Autodesk Inventor part; units mm, degrees
ref_plane "YZ Plane" through (0, 0, 0) normal (1, 0, 0) x (0, 1, 0)
ref_plane "XZ Plane" through (0, 0, 0) normal (0, 1, 0) x (-1, 0, 0)
ref_plane "XY Plane" through (0, 0, 0) normal (0, 0, 1) x (1, 0, 0)
sketch "Sketch1" plane through (0, 0, 0) normal (0, 1, 0) x (-1, 0, 0)
  line L0 (-5.5, -12) -> (5.5, -12)
  line L1 (5.5, -12) -> (5.5, 12)
  line L2 (5.5, 12) -> (-5.5, 12)
  line L3 (-5.5, 12) -> (-5.5, -12)
  line L4 (-5.5, -12) -> (5.5, 12) construction
  line L5 (5.5, -12) -> (-5.5, 12) construction
  point P0 (0, 0)
  dimension "d0" = 11
  dimension "d1" = 24
extrude "Extrusion1" add sketch "Sketch1" along normal blind 10
shell "Shell1" thickness 1 removed faces 1 at (1.8333, 10, 4)
sketch "Sketch2" plane through (-5.5, 0, 12) normal (0, 0, 1) x (1, 0, 0)
  line L0 (0, 10) -> (11, 10)
  circle A0 centre (5.5, 6.75) radius 3.5
  point P0 (5.5, 0)
  point P1 (4.201, 10)
  point P2 (6.799, 10)
  dimension "d5" = 7
  dimension "d6" = 0.25
extrude "Extrusion2" cut sketch "Sketch2" against normal blind 9 contours L0 A0 picked at (4.7002, 5.9949)
sketch "Sketch3" plane through (0, 10, 0) normal (0, 1, 0) x (1, 0, 0)
  line L0 (1.299, -12) -> (5.5, -12)
  line L1 (5.5, -12) -> (5.5, 12)
  line L2 (5.5, 12) -> (-5.5, 12)
  line L3 (-5.5, 12) -> (-5.5, -12)
  line L4 (-5.5, -12) -> (-1.299, -12)
  line L5 (-5.5, 12) -> (5.5, 12)
  line L6 (5.5, 12) -> (5.5, -12)
  line L7 (5.5, -12) -> (-5.5, -12)
  line L8 (-5.5, -12) -> (-5.5, 12)
  point P0 (0, 0)
  point P1 (-1.299, -12)
extrude "Extrusion3" add sketch "Sketch3" along normal blind 1
sketch "Sketch5" plane through (0, 0, 0) normal (0, -1, 0) x (1, 0, 0)
  line L0 (4.5, -11) -> (-4.5, -11)
  line L1 (3, -11) -> (-3, -11)
  line L2 (-3, -11) -> (-3, -6.5)
  line L3 (-2.25, -5.75) -> (2.25, -5.75)
  line L4 (3, -6.5) -> (3, -11)
  arc A0 (3, -6.5) -> (2.25, -5.75) centre (2.25, -6.5) ccw
  arc A1 (-2.25, -5.75) -> (-3, -6.5) centre (-2.25, -6.5) ccw
  line L5 (-5.5, -12) -> (-5.5, 12)
  line L6 (5.5, 12) -> (5.5, -12)
  line L7 (-3, -11) -> (-5.5, -11)
  line L8 (3, -11) -> (5.5, -11)
  point P0 (0, 0)
  point P1 (3, -5.75)
  dimension "d19" = 5.25
  dimension "d20" = 0.75
  dimension "d23" = 6
extrude "Extrusion5" cut sketch "Sketch5" against normal blind 10
properties part number "carcasaXeotype_FLEX-SENSOR"
Could you check a few things on this model? Use its own coordinates, in mm. A direction names the side the tool comes from. Coordinates: 2 decimals unless noted, no trailing zeros. Order: outer loops, then holes, each group sorted by start corner. A loop starts at its lowest first (then second) coordinate and runs counter-clockwise, first axis right, second up. Notation, with made-up numbers: M 47.5,-5.75 L 75.5,-5.75 A24 ccw 75.5,32.25 Z; hole C 2,77 d8. An arc over 180 degrees is marked long. Use one line per item in the form item = value. Start each with the question number.
1. Suppose I cut it at D-D on x = 4. Write out the boundary of the cut face in (y, z), then the cut area to 3 significant figures.
2. Suppose I cut it at C-C on z = -1.5. Write out the boundary of the cut face in (x, y).
3. Suppose I cut it at B-B on y = 6.75. Write out the boundary of the cut face in (x, z).
4. On a 3-axis mill with a long thin cutter (end or side, diameter ignored), from which of +Z, -Z, +X, -X, +Y, -Y can I reach the whole of each face in a straight line? I mean faces 4 (the flat face through (0, 0.5, -5.75)), 5 (the flat face through (0, 5, -12)), 6 (the flat face through (0, 5, -11)), 7 (the flat face through (-5.5, 5, 0)), 8 (the cylindrical face through (-0.135, 3.253, 11.507)). Say none if no direction works.
5. We'd pull the mould along Y, two halves only. Please class faces 1 (the flat face through (0, 10, 0)), 2 (the flat face through (-3, 0.5, -8.8)), 3 (the flat face through (0, 0, 0)): +Y half, -Y half, draft (parallel to the pull), parting line (faces both ways), or undercut.
6. Please list where these lines run through material, in increasing order: line 1 (X direction, y = 3.5, z = 3.5); line 2 (Y direction, x = 0, z = 11.7); line 3 (Y direction, x = -1.25, z = 4.5).
7. Suppose I cut it at A-A on x = 0. Write out the boundary of the cut face in (y, z).
8. For pin 1 (6 mm diameter, centred on x = -2.5, z = 0, fed in from -Y); pin 2 (2.5 mm diameter, centred on x = 0.5, y = 7.5, fed in from +Z), each with a flat end and sliding along its axis, tell me the tip position at first contact or that it passes through.
Geometry says:
q1.outline = M 0,-12 L 11,-12 L 11,12 L 0,12 Z; hole M 1,-11 L 10,-11 L 10,11 L 1,11 Z
q1.area = 66.0 mm^2
q2.outline = M -5.5,0 L 5.5,0 L 5.5,11 L -5.5,11 Z; hole M -4.5,1 L 4.5,1 L 4.5,10 L -4.5,10 Z
q3.outline = M -5.5,-12 L 5.5,-12 L 5.5,12 L 3.5,12 L 3.5,11 L 4.5,11 L 4.5,-11 L -4.5,-11 L -4.5,11 L -3.5,11 L -3.5,12 L -5.5,12 Z
q4.face_4 = -Y
q4.face_5 = -Z, +X, -X, +Y, -Y
q4.face_6 = none
q4.face_7 = +Z, -Z, -X, +Y, -Y
q4.face_8 = +Z
q5.face_1 = undercut
q5.face_2 = draft
q5.face_3 = -Y half
q6.line_1 = -5.5 to -4.5, 4.5 to 5.5
q6.line_2 = 0 to 3.25, 10 to 11
q6.line_3 = 0 to 1, 10 to 11
q7.outline = M 0,-12 L 11,-12 L 11,12 L 10,12 L 10,-11 L 0,-11 Z; M 0,-5.75 L 1,-5.75 L 1,11 L 3.25,11 L 3.25,12 L 0,12 Z
q8.pin_1 = 0
q8.pin_2 = -11
